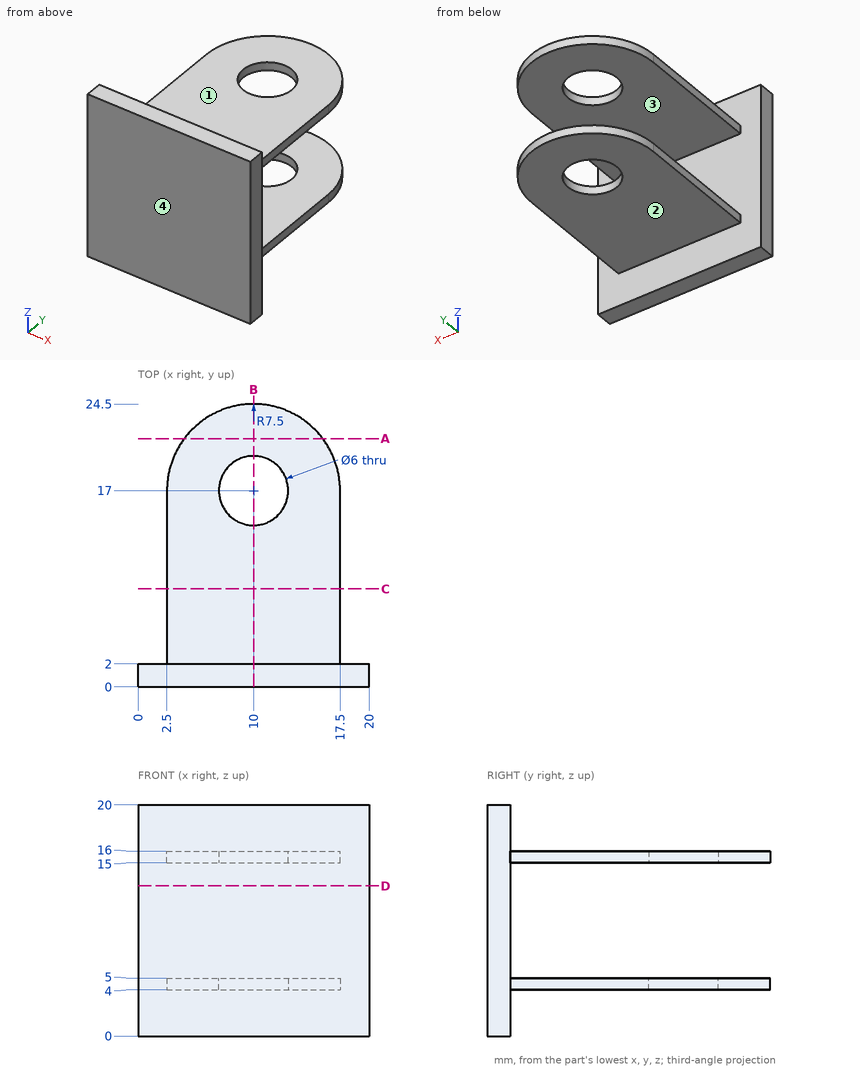
The figure shows three views and two pictorial views of one solid part (mm, origin at its lowest corner). Answer the questions. A direction names the side the tool comes from. Coordinates: 2 decimals unless noted, no trailing zeros. Loops run counter-clockwise (first coordinate to the right, second up) from the corner with the lowest first, then second, coordinate; pieces in that order, holes last. Notation, with made-up numbers: (89.5, 43.5) -> (103.5, 43.5) arc R21 cw to (103.5, 52.5) -> close; hole circle Ø7 at (37, 43). An arc over 180 degrees is marked (long way). Use one line per item in the form item = value. Start each with the question number.
Item 1: The part is cut by section A-A on y = 21.5. Determine the outline of the cut face in (x, z), then the cut area to 3 significant figures.
Item 2: Flat-ended cylindrical pins translate along their axes: pin 1 Ø12 at (x, y) = (12, 10.5) entering from +Z; pin 2 Ø0.5 at (y, z) = (11.5, 4.5) entering from -X; pin 3 Ø6 at (x, z) = (12.5, 17.5) entering from -Y; pin 4 Ø8 at (x, z) = (2.5, 10) entering from +Y. Find the tip coordinate at first contact, or state that the pin passes through.
Item 3: The part is cut by section C-C on y = 8.5. Determine the outline of the cut face in (x, z), then the cut area to 3 significant figures.
Item 4: Consider L1, parallel to Z at x = 5, y = 8; L2, parallel to Y at x = 10, z = 15.75; L3, parallel to Y at x = 1, z = 9. Determine where each line is inside the solid, lowest interval first. Write a range as [from, to].
Item 5: A tool of negligible diameter and unlimited length cuts with its end or side. For the marked faces 1, 2, 3 and 4, from which of +Z, -Z, +X, -X, +Y, -Y can it reach the whole face along a straight path? Write none if from no direction.
Item 6: The part is cut by section D-D on z = 13. Determine the outline of the cut face in (x, y).
Item 7: The part is cut by section B-B on x = 10. Determine the outline of the cut face in (y, z).
Answer key:
q1.outline = (4, 4) -> (16, 4) -> (16, 5) -> (4, 5) -> close; (4, 15) -> (16, 15) -> (16, 16) -> (4, 16) -> close
q1.area = 24.0 mm2
q2.pin_1 = 16
q2.pin_2 = 2.5
q2.pin_3 = 0
q2.pin_4 = 2
q3.outline = (2.5, 4) -> (17.5, 4) -> (17.5, 5) -> (2.5, 5) -> close; (2.5, 15) -> (17.5, 15) -> (17.5, 16) -> (2.5, 16) -> close
q3.area = 30.0 mm2
q4.L1 = [4, 5], [15, 16]
q4.L2 = [0, 14], [20, 24.5]
q4.L3 = [0, 2]
q5.face_1 = +Z, +X, -X, +Y
q5.face_2 = -Z, +X, -X, +Y
q5.face_3 = +X, -X, +Y
q5.face_4 = +Z, -Z, +X, -X, -Y
q6.outline = (0, 0) -> (20, 0) -> (20, 2) -> (0, 2) -> close
q7.outline = (0, 0) -> (2, 0) -> (2, 4) -> (14, 4) -> (14, 5) -> (2, 5) -> (2, 15) -> (14, 15) -> (14, 16) -> (2, 16) -> (2, 20) -> (0, 20) -> close; (20, 4) -> (24.5, 4) -> (24.5, 5) -> (20, 5) -> close; (20, 15) -> (24.5, 15) -> (24.5, 16) -> (20, 16) -> close
